CAD build for the part. Positions are in the model's coordinates, mm. A direction names the side the tool comes from. Give positions to 0.01 mm unless a question says otherwise; leave off trailing zeros. Write each loop counter-clockwise with the first axis right and the second up, starting at its lowest first coordinate (ties: lowest second). Pieces come first, ordered by that corner, then holes. Notation, with made-up numbers: (45, 65.25) -> (74, 65.25) arc R28 cw to (74, 95.25) -> close; hole circle Ø3 at (84, 6). An arc over 180 degrees is marked (long way). Answer in a Markdown table with one row per item. Add a question column.
```python
from build123d import *

# Parameters (mm, degrees)
SKETCH1_R           = 1.55
SKETCH1_R_2         = 1.45
BOSS_EXTRUDE1_DEPTH = 4.75
FILLET2_R           = 1
CUT_EXTRUDE1_DEPTH  = 3
BOSS_EXTRUDE2_DEPTH = 2.75
CUT_EXTRUDE2_DEPTH  = 3
SKETCH7_R           = 0.95
CUT_EXTRUDE3_DEPTH  = 51.921508226


with BuildPart() as part:
    # Sketch1 → Boss-Extrude1 (new body)
    with BuildSketch(Plane.XY):
        with BuildLine():
            Line((-8, 0), (-8, 40))
            ThreePointArc((-8, 40), (0, 48), (8, 40))
            Line((8, 40), (8, 0))
            ThreePointArc((8, 0), (0, -8), (-8, 0))
        make_face()
        with Locations((0, 40)):
            Circle(SKETCH1_R, mode=Mode.SUBTRACT)
        Circle(SKETCH1_R, mode=Mode.SUBTRACT)
        with Locations((5.258025032, 10)):
            Circle(SKETCH1_R_2, mode=Mode.SUBTRACT)
    extrude(amount=BOSS_EXTRUDE1_DEPTH)

    # Fillet2
    fillet2_edges = [part.edges().sort_by_distance(p)[0] for p in [
        (0, 48, 4.75),
        (-8, 20, 4.75),
        (0, -8, 4.75),
        (8, 20, 4.75),
    ]]
    fillet(fillet2_edges, radius=FILLET2_R)

    # Sketch2 → Cut-Extrude1 (cut)
    with BuildSketch(Plane.XY.offset(4.75)):
        Polygon((3.175426481, 40), (1.58771324, 42.75), (-1.58771324, 42.75), (-3.175426481, 40), (-1.58771324, 37.25), (1.58771324, 37.25), align=None)
        Polygon((3.175426481, 0), (1.58771324, 2.75), (-1.58771324, 2.75), (-3.175426481, 0), (-1.58771324, -2.75), (1.58771324, -2.75), align=None)
    extrude(amount=-CUT_EXTRUDE1_DEPTH, mode=Mode.SUBTRACT)

    # Sketch3 → Boss-Extrude2 (add)
    with BuildSketch(Plane(origin=(0, 0, 0), x_dir=(-1, 0, 0), z_dir=(0, 0, -1))):
        Polygon((8, 30), (3, 30), (-6.304970195, 30), (0, 14), (3, 12), (8, 12), align=None)
    extrude(amount=BOSS_EXTRUDE2_DEPTH)

    # Mirror5: part across plane


with BuildPart() as part_1:
    add(part.part)
    add(part.part.mirror(Plane.XY.offset(-2.75)))

    # Sketch4 → Cut-Extrude2 (cut)
    with BuildSketch(Plane.XY.offset(-5.5)):
        Polygon((2, 12.305922059), (2, 15.02352233), (8, 36.305922059), (8, 12.305922059), align=None)
    cut_extrude2 = extrude(amount=-CUT_EXTRUDE2_DEPTH, mode=Mode.SUBTRACT)

    # Mirror6: Cut-Extrude2 across plane
    add(cut_extrude2.mirror(Plane(origin=(0, 0, -2.75), x_dir=(1, 0, 0), z_dir=(0, 0, -1))), mode=Mode.SUBTRACT)

    # Sketch7 → Cut-Extrude3 (cut, through all)
    with BuildSketch(Plane(origin=(0, 0, -10.25), x_dir=(-1, 0, 0), z_dir=(0, 0, -1))):
        with Locations((-3.5, 28)):
            Circle(SKETCH7_R)
        with Locations(Location((3.5, 28, 0), (0, 0, 180))):
            Circle(SKETCH7_R)
    extrude(amount=-CUT_EXTRUDE3_DEPTH, mode=Mode.SUBTRACT)


solid = part_1.part
```
Item 1: Slice it at A-A, the plane y = 10. List the corners of the cut face in (x, z), then the cut area to 3 significant figures.
Item 2: Drop flat-ended pins along their axis: pin 1 Ø1.5 at (y, z) = (14, -5) entering from +X; pin 2 Ø4 at (x, y) = (0, 40) entering from -Z; pin 3 Ø5 at (x, z) = (6, -7.5) entering from +Y; pin 4 Ø3 at (x, y) = (0, 40) entering from +Z. Give the stop position or say it passes through.
Item 3: Slice it at C-C, the plane z = -0.5. List the corners of the cut face in (x, y), then the cut area to 3 significant figures.
Item 4: Slice it at D-D, the plane y = 33. List the corners of the cut face in (x, z), then the cut area to 3 significant figures.
Item 5: Which spindle directions (+Z, -Z, +X, -X, +Y, -Y) get a long thin tool onto all of the face, cutting with end or side? Do faces 4 (the face through (2.37, 38.606, 3.271)), 5 (the face through (4.96, 25.52, 1.48)), 6 (the face through (0, -2.75, -9)). Say none if no direction does.
Item 6: Mould opens along Z. For faces 1 (the face through (2, 14, 1)), 2 (the face through (-7.715, 20.28, -9.949)), 3 (the face through (0.715, -1.375, 0.863)) say: released by +Z, released by -Z, zero draft, split by the parting line, or undercut.
Item 7: Probe L1, parallel to Z at x = -0.75, y = 6; L2, parallel to Z at x = 4.25, y = 19.5; L3, parallel to X at y = 40, z = 1.1. List the from-to ranges inside material, lowest first. Write a range as from..to.
Item 8: Slice it at B-B, the plane z = -6.5. List the corners of the cut face in (x, y), then the cut area to 3 significant figures.
Answer key:
| question | item | result |
|---|---|---|
| 1 | outline | (-8, -9.25) arc R1 ccw to (-7, -10.25) -> (3.81, -10.25) -> (3.81, -5.5) -> (-8, -5.5) -> close; (-8, 0) -> (3.81, 0) -> (3.81, 4.75) -> (-7, 4.75) arc R1 ccw to (-8, 3.75) -> close; (6.71, -10.25) -> (7, -10.25) arc R1 ccw to (8, -9.25) -> (8, -5.5) -> (6.71, -5.5) -> close; (6.71, 0) -> (8, 0) -> (8, 3.75) arc R1 ccw to (7, 4.75) -> (6.71, 4.75) -> close |
| 1 | area | 124 mm² |
| 2 | pin 1 | stops at x = 2 |
| 2 | pin 2 | stops at z = -7.25 |
| 2 | pin 3 | stops at y = 47.19 |
| 2 | pin 4 | passes through |
| 3 | outline | (-8, 12) -> (-3, 12) -> (0, 14) -> (6.3, 30) -> (-8, 30) -> close; hole circle Ø1.9 at (-3.5, 28); hole circle Ø1.9 at (3.5, 28) |
| 3 | area | 186 mm² |
| 4 | outline | (-8, -9.25) arc R1 ccw to (-7, -10.25) -> (7, -10.25) arc R1 ccw to (8, -9.25) -> (8, -8.5) -> (7.07, -8.5) -> (7.07, -5.5) -> (-8, -5.5) -> close; (-8, 0) -> (7.07, 0) -> (7.07, 3) -> (8, 3) -> (8, 3.75) arc R1 ccw to (7, 4.75) -> (-7, 4.75) arc R1 ccw to (-8, 3.75) -> close |
| 4 | area | 146 mm² |
| 5 | face 4 | +Z |
| 5 | face 5 | +X |
| 5 | face 6 | -Z |
| 6 | face 1 | undercut |
| 6 | face 2 | released by -Z |
| 6 | face 3 | zero draft |
| 7 | L1 | z = -10.25..-5.5, 0..4.75 |
| 7 | L2 | z = -10.25..-8.5, 3..4.75 |
| 7 | L3 | x = -8..-1.55, 1.55..8 |
| 8 | outline | (-8, 0) arc R8 ccw to (8, 0) -> (8, 12.31) -> (2, 12.31) -> (2, 15.02) -> (8, 36.31) -> (8, 40) arc R8 ccw to (-8, 40) -> close; hole circle Ø1.9 at (-3.5, 28); hole circle Ø3.1 at (0, 0); hole circle Ø3.1 at (0, 40); hole circle Ø1.9 at (3.5, 28); hole circle Ø2.9 at (5.26, 10) |
| 8 | area | 734 mm² |
